```python
from build123d import *

# Parameters (mm, degrees)
ESQUISSE1_R             = 26
ESQUISSE1_R_2           = 16
BOSS_EXTRU_1_DEPTH      = 10
ESQUISSE2_R             = 35
BOSS_EXTRU_2_DEPTH      = 5
ESQUISSE3_R             = 16
ENL_V_MAT_EXTRU_1_DEPTH = 5
ESQUISSE4_R             = 1.5
ENL_V_MAT_EXTRU_2_DEPTH = 35
ENL_V_MAT_EXTRU_3_DEPTH = 3


with BuildPart() as part:
    # Esquisse1 → Boss.-Extru.1 (new body)
    with BuildSketch(Plane(origin=(0, 0, 0), x_dir=(1, 0, 0), z_dir=(0, 1, 0))):
        Circle(ESQUISSE1_R)
        Circle(ESQUISSE1_R_2, mode=Mode.SUBTRACT)
    extrude(amount=BOSS_EXTRU_1_DEPTH)

    # Esquisse2 → Boss.-Extru.2 (add)
    with BuildSketch(Plane.XZ):
        Circle(ESQUISSE2_R)
    extrude(amount=-BOSS_EXTRU_2_DEPTH)

    # Esquisse3 → Enlèv. mat.-Extru.1 (cut)
    with BuildSketch(Plane(origin=(0, 5, 0), x_dir=(1, 0, 0), z_dir=(0, 1, 0))):
        Circle(ESQUISSE3_R)
    extrude(amount=-ENL_V_MAT_EXTRU_1_DEPTH, mode=Mode.SUBTRACT)

    # Esquisse4 → Enlèv. mat.-Extru.2 (cut)
    with BuildSketch(Plane(origin=(0, 10, 0), x_dir=(1, 0, 0), z_dir=(0, 1, 0))):
        with Locations((-21, 0)):
            Circle(ESQUISSE4_R)
        with Locations((21, 0)):
            Circle(ESQUISSE4_R)
        with Locations((0, -21)):
            Circle(ESQUISSE4_R)
        with Locations((0, 21)):
            Circle(ESQUISSE4_R)
    extrude(amount=-ENL_V_MAT_EXTRU_2_DEPTH, mode=Mode.SUBTRACT)

    # Esquisse5 → Enlèv. mat.-Extru.3 (cut)
    with BuildSketch(Plane.XZ):
        Polygon((24.031088913, 0), (22.515544457, 2.625), (19.484455543, 2.625), (17.968911087, 0), (19.484455543, -2.625), (22.515544457, -2.625), align=None)
        Polygon((3.031088913, -21), (1.515544457, -18.375), (-1.515544457, -18.375), (-3.031088913, -21), (-1.515544457, -23.625), (1.515544457, -23.625), align=None)
        Polygon((-17.968911087, 0), (-19.484455543, 2.625), (-22.515544457, 2.625), (-24.031088913, 0), (-22.515544457, -2.625), (-19.484455543, -2.625), align=None)
        Polygon((3.031088913, 21), (1.515544457, 23.625), (-1.515544457, 23.625), (-3.031088913, 21), (-1.515544457, 18.375), (1.515544457, 18.375), align=None)
    extrude(amount=-ENL_V_MAT_EXTRU_3_DEPTH, mode=Mode.SUBTRACT)


solid = part.part
```
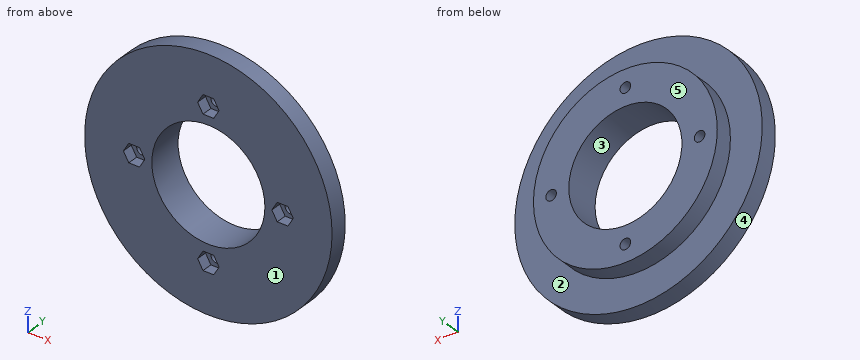
Part model, mm, in its own coordinate system. Face numbers are marked on the shaded views. A direction names the side the tool comes from. Coordinates: 2 decimals unless noted, no trailing zeros. Order: outer loops, then holes, each group sorted by start corner. A loop starts at its lowest first (then second) coordinate and runs counter-clockwise, first axis right, second up. Notation, with made-up numbers: (30, 72) -> (53, 72) arc R7 cw to (53, 85) -> close; hole circle Ø4 at (65, -20.5). An arc over 180 degrees is marked (long way). Put each result on its own line as item: value. Start each with the question number.
(1) Mould opens along Z. For the marked faces 3, 4 and 5 say: pulls with the +Z half, pulls with the -Z half, needs draft (parallel to the pull), parting line crosses it, or undercut.
(2) Band-saw the part on C-C (y = 4). Give the cut face in (x, z), then the cut area to 3 significant figures.
(3) Band-saw the part on A-A (x = 0). Give the cut face in (y, z) (3 decimals), then the cut area to 4 significant figures.
(4) Band-saw the part on D-D (z = -11). Give the cut face in (x, y), then the cut area to 3 significant figures.
(5) Pin check, flat tips, straight feed: pin 1 Ø4 at (x, y) = (-16.5, 5) entering from +Z; pin 2 Ø2.5 at (x, y) = (0.5, 1) entering from -Z; pin 3 Ø2.5 at (x, z) = (0, 21) entering from -Y; pin 4 Ø0.9 at (x, y) = (0, 2) entering from +Z. Stop position of each tip, or through.
(6) Which spindle directions (+Z, -Z, +X, -X, +Y, -Y) get a long thin tool onto all of the face, cutting with end or side? Do the marked faces 1 and 2. Say none if no direction does.
(7) Band-saw the part on B-B (x = -8.5). Give the cut face in (y, z).
(8) Probe line 1 along Z through (x, y) = (0, 7.75); line 2 along Z through (x, y) = (0, 2) (3 decimals); line 3 along X through (y, z) = (6.5, 21). List the from-to ranges inside material, lowest first. Write a range as [from, to].
Determined:
1. face 3: undercut
1. face 4: parting line crosses it
1. face 5: needs draft
2. outline: circle Ø70 at (0, 0); hole circle Ø3 at (-21, 0); hole circle Ø32 at (0, 0); hole circle Ø3 at (0, -21); hole circle Ø3 at (0, 21); hole circle Ø3 at (21, 0)
2. area: 3,020 mm²
3. outline: (0, -35) -> (5, -35) -> (5, -26) -> (10, -26) -> (10, -22.5) -> (3, -22.5) -> (3, -23.625) -> (0, -23.625) -> close; (0, -18.375) -> (3, -18.375) -> (3, -19.5) -> (10, -19.5) -> (10, -16) -> (0, -16) -> close; (0, 16) -> (10, 16) -> (10, 19.5) -> (3, 19.5) -> (3, 18.375) -> (0, 18.375) -> close; (0, 23.625) -> (3, 23.625) -> (3, 22.5) -> (10, 22.5) -> (10, 26) -> (5, 26) -> (5, 35) -> (0, 35) -> close
3. area: 216.5 mm²
4. outline: (-33.23, 0) -> (-11.62, 0) -> (-11.62, 10) -> (-23.56, 10) -> (-23.56, 5) -> (-33.23, 5) -> close; (11.62, 0) -> (33.23, 0) -> (33.23, 5) -> (23.56, 5) -> (23.56, 10) -> (11.62, 10) -> close
4. area: 335 mm²
5. pin 1: stops at z = 31.86
5. pin 2: stops at z = -35
5. pin 3: passes through
5. pin 4: stops at z = 35
6. face 1: +Z, -Z, +X, -X, -Y
6. face 2: +Y
7. outline: (0, -33.95) -> (5, -33.95) -> (5, -24.57) -> (10, -24.57) -> (10, -13.56) -> (0, -13.56) -> close; (0, 13.56) -> (10, 13.56) -> (10, 24.57) -> (5, 24.57) -> (5, 33.95) -> (0, 33.95) -> close
8. line 1: z = [-26, -22.5], [-19.5, -16], [16, 19.5], [22.5, 26]
8. line 2: z = [-35, -23.625], [-18.375, -16], [16, 18.375], [23.625, 35]
8. line 3: x = [-15.33, -1.5], [1.5, 15.33]
